from build123d import *

# Parameters (mm, degrees)
SKETCH1_R           = 3.1
BOSS_EXTRUDE1_DEPTH = 3
BOSS_EXTRUDE2_START = 0.5
BOSS_EXTRUDE2_DEPTH = 0.5
SKETCH3_R           = 0.85
CUT_EXTRUDE1_DEPTH  = 2.5
SKETCH4_R           = 1
CUT_EXTRUDE2_DEPTH  = 12.324751653


with BuildPart() as part:
    # Sketch1 → Boss-Extrude1 (new body)
    with BuildSketch(Plane(origin=(0, 0, 0), x_dir=(1, 0, 0), z_dir=(0, 1, 0))):
        with BuildLine():
            Line((4, 6), (4, -6))
            ThreePointArc((4, -6), (0, -10), (-4, -6))
            Line((-4, -6), (-4, 6))
            ThreePointArc((-4, 6), (0, 10), (4, 6))
        make_face()
        with Locations(Location((0, 6, 0), (0, 0, 270))):
            Circle(SKETCH1_R, mode=Mode.SUBTRACT)
        with Locations(Location((0, -6, 0), (0, 0, 270))):
            Circle(SKETCH1_R, mode=Mode.SUBTRACT)
    extrude(amount=BOSS_EXTRUDE1_DEPTH)

    # Sketch2 → Boss-Extrude2 (add)
    with BuildSketch(Plane.XZ.offset(BOSS_EXTRUDE2_START)):
        with BuildLine():
            Line((4, 6), (4, -6))
            ThreePointArc((4, -6), (0, -10), (-4, -6))
            Line((-4, -6), (-4, 6))
            ThreePointArc((-4, 6), (0, 10), (4, 6))
        make_face()
    extrude(amount=-BOSS_EXTRUDE2_DEPTH)

    # Sketch3 → Cut-Extrude1 (cut)
    with BuildSketch(Plane.XZ.offset(0.5)):
        with Locations(Location((0, 0, 0), (0, 0, 270))):
            Circle(SKETCH3_R)
    extrude(amount=-CUT_EXTRUDE1_DEPTH, mode=Mode.SUBTRACT)

    # Sketch4 → Cut-Extrude2 (cut, through all)
    with BuildSketch(Plane.XZ.offset(0.5)):
        with Locations(Location((0, 6, 0), (0, 0, 270))):
            Circle(SKETCH4_R)
        with Locations(Location((0, -6, 0), (0, 0, 270))):
            Circle(SKETCH4_R)
    extrude(amount=-CUT_EXTRUDE2_DEPTH, mode=Mode.SUBTRACT)


solid = part.part
The model under review builds one solid part; all positions refer to its coordinate system, in mm. A direction names the side the tool comes from. Coordinates: 2 decimals unless noted, no trailing zeros. Loops run counter-clockwise (first coordinate to the right, second up) from the corner with the lowest first, then second, coordinate; pieces in that order, holes last. Notation, with made-up numbers: (18, -23.75) -> (67, -23.75) arc R24 ccw to (67, -7.75) -> close; hole circle Ø6 at (89, 12.5). An arc over 180 degrees is marked (long way). Use a Markdown table: item, result. Add a question column.
1. Add section D-D on y = 0.75. Write out the cut boundary in (x, z), plus the area to 3 significant figures.
2. Machinability: for faces 1 (the face through (-0.6, -0.3, 6.8)), 2 (the face through (0, 2, 0)), 3 (the face through (1, 0, -5)), which of the approach directions +Z, -Z, +X, -X, +Y, -Y give a long, thin tool a straight path to every point of the face, cutting with its end or side? Answer none if there is none.
3. Add section C-C on y = 2.5. Write out the cut boundary in (x, z).
4. Clearance check with flat-ended pins moving along their axes: pin 1 Ø2.5 at (x, z) = (0, -6) entering from -Y; pin 2 Ø1.5 at (x, z) = (0.5, -5) entering from +Y. State where each tip first meets the part, or that it passes through.
5. Draft analysis for pull direction Z (two halves, no side actions). For faces 4 (the face through (1, 0, 7)), 5 (the face through (0, 3, 0)), 6 (the face through (0, 1, 10)), state which applies: pulls with the +Z half, pulls with the -Z half, needs draft (parallel to the pull), parting line crosses it, or undercut.
6. Add section A-A on x = 0. Write out the cut boundary in (y, z), plus the area to 4 significant figures.
7. To check wall thickness, follow line 1 (X direction, y = 2.45, z = -6); line 2 (Z direction, x = -0.75, y = -0.3); line 3 (Z direction, x = -2.75, y = 1.5). State the ranges of each line that lie inside material, in increasing order.
8. Add section B-B on z = 0. Write out the cut boundary in (x, y).
Returned:
| question | item | result |
|---|---|---|
| 1 | outline | (-4, -6) arc R4 ccw to (4, -6) -> (4, 6) arc R4 ccw to (-4, 6) -> close; hole circle Ø6.2 at (0, -6); hole circle Ø6.2 at (0, 6); hole circle Ø1.7 at (0, 0) |
| 1 | area | 83.6 mm² |
| 2 | face 1 | +Y, -Y |
| 2 | face 2 | -Y |
| 2 | face 3 | +Y |
| 3 | outline | (-4, -6) arc R4 ccw to (4, -6) -> (4, 6) arc R4 ccw to (-4, 6) -> close; hole circle Ø6.2 at (0, -6); hole circle Ø6.2 at (0, 6) |
| 4 | pin 1 | stops at y = -0.5 |
| 4 | pin 2 | stops at y = 0 |
| 5 | face 4 | undercut |
| 5 | face 5 | needs draft |
| 5 | face 6 | pulls with the +Z half |
| 6 | outline | (-0.5, -10) -> (3, -10) -> (3, -9.1) -> (0, -9.1) -> (0, -7) -> (-0.5, -7) -> close; (-0.5, -5) -> (0, -5) -> (0, -2.9) -> (3, -2.9) -> (3, 2.9) -> (0, 2.9) -> (0, 5) -> (-0.5, 5) -> (-0.5, 0.85) -> (2, 0.85) -> (2, -0.85) -> (-0.5, -0.85) -> close; (-0.5, 7) -> (0, 7) -> (0, 9.1) -> (3, 9.1) -> (3, 10) -> (-0.5, 10) -> close |
| 6 | area | 26.55 mm² |
| 7 | line 1 | x = -4 to -3.1, 3.1 to 4 |
| 7 | line 2 | z = -9.93 to -6.66, -5.34 to -0.4, 0.4 to 5.34, 6.66 to 9.93 |
| 7 | line 3 | z = -8.9 to -7.43, -4.57 to 4.57, 7.43 to 8.9 |
| 8 | outline | (-4, -0.5) -> (-0.85, -0.5) -> (-0.85, 2) -> (0.85, 2) -> (0.85, -0.5) -> (4, -0.5) -> (4, 3) -> (-4, 3) -> close |
